Here's the drawing with two shaded views (mm, measured from the low corner). I have some questions. Coordinates: 2 decimals unless noted, no trailing zeros. Order: outer loops, then holes, each group sorted by start corner. A loop starts at its lowest first (then second) coordinate and runs counter-clockwise, first axis right, second up. Notation, with made-up numbers: (17.25, 25) - (45.25, 25) arc R25 ccw to (45.25, 63) - close; hole circle Ø9 at (-3, 60.5). An arc over 180 degrees is marked (long way). Answer as CSV lines item,"result". Start each with the question number.
1. I need wall thicknesses on probe 1 along Y at (x, z) = (7.5, 0.3); probe 2 along X at (y, z) = (73.5, 0.3); probe 3 along X at (y, z) = (43, 0.25). Which ranges of each line are inside material? Lowest first, please.
2. I want a section at C-C, the plane x = 70. List the corners of the cut face in (y, z) for me.
3. I want a section at A-A, the plane y = 40. List the corners of the cut face in (x, z) for me, and give its area (3 significant figures).
4. I want a section at D-D, the plane z = 1.2. List the corners of the cut face in (x, y) for me.
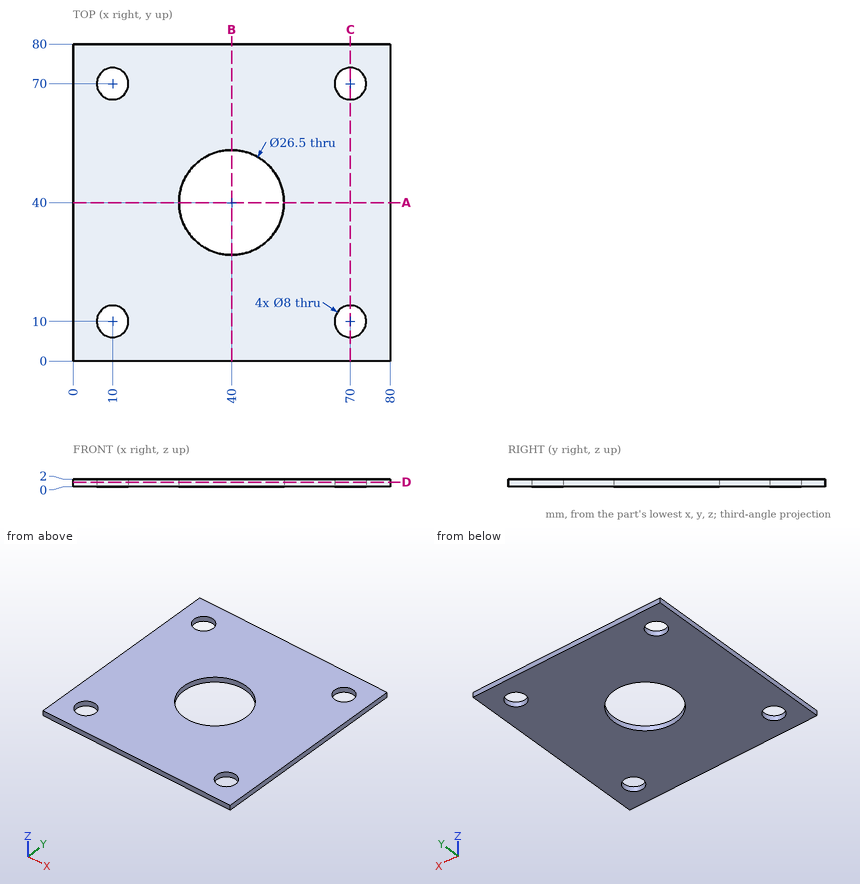
Solved:
1,probe 1,"y = 0 to 6.88, 13.12 to 66.88, 73.12 to 80"
1,probe 2,"x = 0 to 8.06, 11.94 to 68.06, 71.94 to 80"
1,probe 3,"x = 0 to 27.09, 52.91 to 80"
2,outline,"(0, 0) - (6, 0) - (6, 2) - (0, 2) - close; (14, 0) - (66, 0) - (66, 2) - (14, 2) - close; (74, 0) - (80, 0) - (80, 2) - (74, 2) - close"
3,outline,"(0, 0) - (26.75, 0) - (26.75, 2) - (0, 2) - close; (53.25, 0) - (80, 0) - (80, 2) - (53.25, 2) - close"
3,area,"107 mm2"
4,outline,"(0, 0) - (80, 0) - (80, 80) - (0, 80) - close; hole circle Ø8 at (10, 10); hole circle Ø8 at (10, 70); hole circle Ø26.5 at (40, 40); hole circle Ø8 at (70, 10); hole circle Ø8 at (70, 70)"
